```python
from build123d import *

# Parameters (mm, degrees)
PAD_DEPTH   = 14
FILLET001_R = 4
FILLET002_R = 16
FILLET_R    = 7


with BuildPart() as part:
    # Sketch → Pad (new body)
    with BuildSketch(Plane.XY):
        with BuildLine():
            Line((-35, -53.5), (-35, -69.5))
            Line((-35, -69.5), (-4.5, -97.94171))
            Line((-4.5, -97.94171), (4.5, -97.94171))
            Line((4.5, -97.94171), (35, -69.5))
            Line((35, -69.5), (35, -53.5))
            Line((35, 33.5), (35, -53.5))
            ThreePointArc((35, 33.5), (29.142136, 47.642136), (15, 53.5))
            Line((-15, 53.5), (15, 53.5))
            ThreePointArc((-15, 53.5), (-29.142136, 47.642136), (-35, 33.5))
            Line((-35, 33.5), (-35, -53.5))
        make_face()
    extrude(amount=PAD_DEPTH)

    # Fillet001
    fillet001_edges = [part.edges().sort_by_distance(p)[0] for p in [
        (-4.5, -97.94171, 7),
        (4.5, -97.94171, 7),
    ]]
    fillet(fillet001_edges, radius=FILLET001_R)

    # Fillet002
    fillet002_edges = [part.edges().sort_by_distance(p)[0] for p in [
        (35, -69.5, 7),
        (-35, -69.5, 7),
    ]]
    fillet(fillet002_edges, radius=FILLET002_R)

    # Fillet
    fillet_edges = [part.edges().sort_by_distance(p)[0] for p in [
        (-17.782163, -85.555893, 14),
        (-33.672961, -68.922987, 14),
        (-4.390363, -97.66338, 14),
        (-35, -58.021501, 14),
        (0, -97.94171, 14),
        (-35, -10, 14),
        (4.390363, -97.66338, 14),
        (-29.142136, 47.642136, 14),
        (17.782163, -85.555893, 14),
        (0, 53.5, 14),
        (33.672961, -68.922987, 14),
        (29.142136, 47.642136, 14),
        (35, -58.021501, 14),
        (35, -10, 14),
    ]]
    fillet(fillet_edges, radius=FILLET_R)


with BuildPart() as part_1:
    # Body104 placement: moved
    add(part.part.moved(Location((0, 0, -0.1))))


solid = part_1.part
```
The listing builds one solid part. Answer for the finished solid, in the listing's coordinates (mm). Round coordinates to 2 decimals unless told otherwise and drop trailing zeros. Loops run counter-clockwise (first coordinate to the right, second up) from the corner with the lowest first, then second, coordinate; pieces in that order, holes last. Notation, with made-up numbers: (12.25, 50.5) -> (45.25, 50.5) arc R33 cw to (45.25, 87.5) -> close; hole circle Ø3 at (56, -0.5). An arc over 180 degrees is marked (long way). Use one line per item in the form item = value.
1. The part is cut by section A-A on z = 1.5. Determine the outline of the cut face in (x, y).
Answer key:
outline = (-35, -62.54) arc R16 ccw to (-29.91, -74.24) -> (-5.65, -96.87) arc R4 ccw to (-2.92, -97.94) -> (2.92, -97.94) arc R4 ccw to (5.65, -96.87) -> (29.91, -74.24) arc R16 ccw to (35, -62.54) -> (35, 33.5) arc R20 ccw to (15, 53.5) -> (-15, 53.5) arc R20 ccw to (-35, 33.5) -> close
2. The part is cut by section B-B on y = -32. Determine the outline of the cut face in (x, z).
Answer key:
outline = (-35, -0.1) -> (35, -0.1) -> (35, 6.9) arc R7 ccw to (28, 13.9) -> (-28, 13.9) arc R7 ccw to (-35, 6.9) -> close
3. Find the intervals of material crossed by probe 1 along X at (y, z) = (-76, 3.75); probe 2 along X at (y, z) = (-68, 13); probe 3 along Y at (x, z) = (20.5, 2.25), in increasing order. Write a range as [from, to].
Answer key:
probe_1 = [-28.03, 28.03]
probe_2 = [-30.17, 30.17]
probe_3 = [-83.02, 52.73]
4. Flat-ended cylindrical pins translate along their axes: pin 1 Ø4 at (x, z) = (23, 2) entering from +Y; pin 2 Ø2 at (y, z) = (-39.5, 8.5) entering from -X; pin 3 Ø1 at (x, z) = (-18, 1.5) entering from -Y. Find the tip coordinate at first contact, or state that the pin passes through.
Answer key:
pin_1 = 52.58
pin_2 = -34.97
pin_3 = -85.82
